Could you check a few things on this model? Use its own coordinates, in mm. A direction names the side the tool comes from. Give positions to 0.01 mm unless a question says otherwise; leave off trailing zeros. Write each loop counter-clockwise with the first axis right and the second up, starting at its lowest first coordinate (ties: lowest second). Pieces come first, ordered by that corner, then holes. Notation, with made-up numbers: (43.5, 63) - (86.5, 63) arc R21 cw to (86.5, 91) - close; hole circle Ø5 at (-2.5, 87.5). An arc over 180 degrees is marked (long way). Answer in a Markdown table with one row per item.
from build123d import *

# Parameters (mm, degrees)
SKETCH1_W                = 31.75
SKETCH1_H                = 84.214152012
BOSS_EXTRUDE1_DEPTH      = 1.905
BOSS_EXTRUDE1_DEPTH_BACK = 46.355
SKETCH3_W                = 12.7
SKETCH3_H                = 52.07
SKETCH3_W_2              = 14.605
SKETCH3_H_2              = 19.05
CUT_EXTRUDE1_DEPTH       = 49.26
CUT_EXTRUDE2_DEPTH       = 65.405
CUT_EXTRUDE3_DEPTH       = 14.605
CUT_EXTRUDE4_REACH       = 67.164
CUT_EXTRUDE5_DEPTH       = 15.24
SKETCH8_R                = 1.016
BOSS_EXTRUDE2_DEPTH      = 5.08
FILLET1_R                = 1.27
FILLET2_R                = 1.27


with BuildPart() as part:
    # Sketch1 → Boss-Extrude1 (new body, two sides)
    with BuildSketch(Plane.XY) as boss_extrude1_sk:
        with Locations((15.875, -42.107076006)):
            Rectangle(SKETCH1_W, SKETCH1_H)
    extrude(amount=BOSS_EXTRUDE1_DEPTH)
    extrude(boss_extrude1_sk.sketch, amount=-BOSS_EXTRUDE1_DEPTH_BACK)

    # Sketch3 → Cut-Extrude1 (cut, through all)
    with BuildSketch(Plane.XY.offset(1.905)):
        with Locations((8.255, -27.94)):
            Rectangle(SKETCH3_W, SKETCH3_H)
        with Locations((7.3025, -74.689152012)):
            Rectangle(SKETCH3_W_2, SKETCH3_H_2)
    extrude(amount=-CUT_EXTRUDE1_DEPTH, mode=Mode.SUBTRACT)

    # Sketch4 → Cut-Extrude2 (cut)
    with BuildSketch(Plane(origin=(0, 0, 0), x_dir=(1, 0, 0), z_dir=(0, 1, 0))):
        Polygon((1.905, 22.225), (1.905, 31.75), (14.405235248, 31.75), (14.405235248, 12.7), (1.905, 12.7), align=None)
    extrude(amount=-CUT_EXTRUDE2_DEPTH, mode=Mode.SUBTRACT)

    # Sketch5 → Cut-Extrude3 (cut)
    with BuildSketch(Plane.ZY):
        Polygon((-22.225, 0), (-12.7, 0), (-12.7, -52.705), (-31.75, -52.705), (-31.75, 0), align=None)
    extrude(amount=-CUT_EXTRUDE3_DEPTH, mode=Mode.SUBTRACT)

    # Sketch6 → Cut-Extrude4 (cut, up to next)
    with BuildSketch(Plane.XZ.offset(65.164152012), mode=Mode.PRIVATE) as cut_extrude4_sk1:
        Polygon((1.905, -22.225), (1.905, 0), (14.605, 0), (14.605, -44.45), (1.905, -44.45), align=None)
    cut_extrude4_tool1 = extrude(cut_extrude4_sk1.sketch, amount=-CUT_EXTRUDE4_REACH, mode=Mode.PRIVATE) & part.part
    add(cut_extrude4_tool1.solids().sort_by_distance((8.255, -65.164152, -22.225))[0], mode=Mode.SUBTRACT)

    # Sketch7 → Cut-Extrude5 (cut)
    with BuildSketch(Plane(origin=(31.75, 0, 0), x_dir=(0, 0, -1), z_dir=(1, 0, 0))):
        Polygon((22.225, -5.08), (35.687, -5.08), (35.687, -55.88), (28.575, -55.88), (28.575, -84.214152012), (15.875, -84.214152012), (15.875, -55.88), (8.763, -55.88), (8.763, -5.08), align=None)
    extrude(amount=-CUT_EXTRUDE5_DEPTH, mode=Mode.SUBTRACT)

    # Sketch8 → Boss-Extrude2 (add)
    with BuildSketch(Plane(origin=(16.51, 0, 0), x_dir=(0, 0, -1), z_dir=(1, 0, 0))):
        with Locations((33.655, -7.62)):
            Circle(SKETCH8_R)
        with Locations((10.795, -7.62)):
            Circle(SKETCH8_R)
    extrude(amount=BOSS_EXTRUDE2_DEPTH)

    # Fillet1
    fillet1_edges = [part.edges().sort_by_distance(p)[0] for p in [
        (24.13, -5.08, -8.763),
        (24.13, -5.08, -35.687),
        (24.13, -55.88, -35.687),
        (24.13, -55.88, -8.763),
    ]]
    fillet(fillet1_edges, radius=FILLET1_R)

    # Fillet2
    fillet2_edges = [part.edges().sort_by_distance(p)[0] for p in [
        (15.875, 0, -46.355),
        (15.875, 0, 1.905),
        (7.3025, -65.164152012, -46.355),
        (7.3025, -65.164152012, 1.905),
    ]]
    fillet(fillet2_edges, radius=FILLET2_R)


solid = part.part
1) If I drill on line 1 (Y direction, x = 20, z = -11); line 2 (Z direction, x = 27.5, y = -58) (3 decimals); line 3 (X direction, y = -31.5, z = -33) (3 decimals), over which ranges is the centre line in solid material (lowest first)?
Check values:
| item | result |
|---|---|
| line 1 | y = -84.21 to -55.88, -8.62 to -6.62, -5.08 to 0 |
| line 2 | z = -46.355 to -28.575, -15.875 to 1.905 |
| line 3 | x = 0 to 1.905, 14.605 to 16.51 |
2) We'd pull the mould along Z, two halves only. Please class faces 1 (the face through (24, -70, -28.575)), 2 (the face through (0, -33, -33)), 3 (the face through (19, -42, -46.355)): +Z half, -Z half, draft (parallel to the pull), parting line (faces both ways), or undercut.
Check values:
| item | result |
|---|---|
| face 1 | undercut |
| face 2 | draft |
| face 3 | -Z half |
3) Imagine slicing it at A-A (y = -45). List the corners of the cut face in (x, z) for me (3 decimals).
Check values:
| item | result |
|---|---|
| outline | (0, -46.355) - (1.905, -46.355) - (1.905, -31.75) - (0, -31.75) - close; (0, -12.7) - (1.905, -12.7) - (1.905, 1.905) - (0, 1.905) - close; (14.605, -46.355) - (31.75, -46.355) - (31.75, -35.687) - (16.51, -35.687) - (16.51, -8.763) - (31.75, -8.763) - (31.75, 1.905) - (14.605, 1.905) - close |
4) Imagine slicing it at B-B (x = 22.5). List the corners of the cut face in (y, z) for me (3 decimals), then the cut area to 3 significant figures.
Check values:
| item | result |
|---|---|
| outline | (-84.214, -46.355) - (-1.27, -46.355) arc R1.27 ccw to (0, -45.085) - (0, 0.635) arc R1.27 ccw to (-1.27, 1.905) - (-84.214, 1.905) - (-84.214, -15.875) - (-55.88, -15.875) - (-55.88, -10.033) arc R1.27 cw to (-54.61, -8.763) - (-6.35, -8.763) arc R1.27 cw to (-5.08, -10.033) - (-5.08, -34.417) arc R1.27 cw to (-6.35, -35.687) - (-54.61, -35.687) arc R1.27 cw to (-55.88, -34.417) - (-55.88, -28.575) - (-84.214, -28.575) - close |
| area | 2,340 mm2 |
5) Will these pins go through, and if not, where does the flat tip stop? P1, Ø0.6, axis at x = 11, z = 1, coming from the +Y side; P2, Ø14, axis at x = 7.5, z = -4.5, coming from the -Y side; P3, Ø1, axis at y = -8, z = -10.5, coming from the +X side; P4, Ø8, axis at y = -43, z = -22.5, coming from the +X side.
Check values:
| item | result |
|---|---|
| P1 | stops at y = 0 |
| P2 | stops at y = -65.16 |
| P3 | stops at x = 21.59 |
| P4 | stops at x = 16.51 |
6) On a 3-axis mill with a long thin cutter (end or side, diameter ignored), from which of +Z, -Z, +X, -X, +Y, -Y can I reach the whole of each face in a straight line? I mean faces 4 (the face through (24, -70, -15.875)), 5 (the face through (8, -60, -44.45)), 6 (the face through (21.59, -8, -11)), 7 (the face through (1, -65.164, -22)). Say none if no direction works.
Check values:
| item | result |
|---|---|
| face 4 | +X, -Y |
| face 5 | -Y |
| face 6 | +X |
| face 7 | +Z, -Z, -X, -Y |
7) Imagine slicing it at D-D (z = -20). List the corners of the cut face in (x, y) for me (3 decimals).
Check values:
| item | result |
|---|---|
| outline | (0, -65.164) - (1.905, -65.164) - (1.905, -52.705) - (0, -52.705) - close; (14.605, -84.214) - (16.51, -84.214) - (16.51, -5.08) - (31.75, -5.08) - (31.75, 0) - (14.605, 0) - close |
8) Imagine slicing it at C-C (y = -61). List the corners of the cut face in (x, z) for me (3 decimals), then the cut area to 3 significant figures.
Check values:
| item | result |
|---|---|
| outline | (0, -46.355) - (31.75, -46.355) - (31.75, -28.575) - (16.51, -28.575) - (16.51, -15.875) - (31.75, -15.875) - (31.75, 1.905) - (0, 1.905) - close; hole (1.905, -44.45) - (14.605, -44.45) - (14.605, 0) - (1.905, 0) - close |
| area | 774 mm2 |
